```python
from build123d import *

# Parameters (mm, degrees)
EXTRUDE_1_DEPTH          = 3
SKETCH_2_R               = 28
EXTRUDE_2_DEPTH          = 3
SKETCH_3_R               = 21.5
CUT_EXTRUDE_1_DEPTH      = 3
FILLET_2_R               = 5
SKETCH_4_R               = 1.275
CUT_EXTRUDE_2_DEPTH      = 4
SKETCH_5_R               = 2.025
CUT_EXTRUDE_3_DEPTH      = 4
SKETCH_6_W               = 25
SKETCH_6_H               = 6
CUT_EXTRUDE_4_DEPTH      = 4
FILLET_3_R               = 2
SKETCH_8_R               = 2.025
CUT_EXTRUDE_5_DEPTH      = 10
SKETCH_9_R               = 2.025
CUT_EXTRUDE_6_DEPTH      = 1
CUT_EXTRUDE_6_DEPTH_BACK = 4
EXTRUDE_3_DEPTH          = 3
FILLET_4_R               = 3


with BuildPart() as part:
    # 草图1 → 凸台-拉伸1 (new body)
    with BuildSketch(Plane.XY):
        Polygon((-35, 0), (0, 0), (0, -30), (25, -30), (25, 20), (-35, 20), align=None)
    extrude(amount=EXTRUDE_1_DEPTH)

    # 草图2 → 凸台-拉伸2 (add)
    with BuildSketch(Plane(origin=(0, 0, 0), x_dir=(-1, 0, 0), z_dir=(0, 0, -1))):
        with Locations((-8.7, 35)):
            Circle(SKETCH_2_R)
    extrude(amount=-EXTRUDE_2_DEPTH)

    # 草图3 → 切除-拉伸1 (cut)
    with BuildSketch(Plane(origin=(0, 0, 0), x_dir=(-1, 0, 0), z_dir=(0, 0, -1))):
        with Locations((-8.7, 35)):
            Circle(SKETCH_3_R)
    extrude(amount=-CUT_EXTRUDE_1_DEPTH, mode=Mode.SUBTRACT)

    # 圆角2
    fillet_2_edges = [part.edges().sort_by_distance(p)[0] for p in [
        (25, 12.233577356, 1.5),
        (-14.943180835, 20, 1.5),
    ]]
    fillet(fillet_2_edges, radius=FILLET_2_R)

    # 草图4 → 切除-拉伸2 (cut, through all)
    with BuildSketch(Plane(origin=(0, 0, 0), x_dir=(-1, 0, 0), z_dir=(0, 0, -1))):
        with Locations((-33.2, 35)):
            Circle(SKETCH_4_R)
        with Locations((-20.95, 56.217622393)):
            Circle(SKETCH_4_R)
        with Locations((3.55, 56.217622393)):
            Circle(SKETCH_4_R)
        with Locations((15.8, 35)):
            Circle(SKETCH_4_R)
        with Locations((3.55, 13.782377607)):
            Circle(SKETCH_4_R)
        with Locations((-20.95, 13.782377607)):
            Circle(SKETCH_4_R)
    extrude(amount=-CUT_EXTRUDE_2_DEPTH, mode=Mode.SUBTRACT)

    # 草图5 → 切除-拉伸3 (cut, through all)
    with BuildSketch(Plane(origin=(0, 0, 0), x_dir=(-1, 0, 0), z_dir=(0, 0, -1))):
        with Locations((-12.5, -8)):
            Circle(SKETCH_5_R)
        with Locations((-12.5, -18)):
            Circle(SKETCH_5_R)
    extrude(amount=-CUT_EXTRUDE_3_DEPTH, mode=Mode.SUBTRACT)

    # 草图6 → 切除-拉伸4 (cut, through all)
    with BuildSketch(Plane(origin=(0, 0, 0), x_dir=(-1, 0, 0), z_dir=(0, 0, -1))):
        with Locations((-12.5, -27)):
            Rectangle(SKETCH_6_W, SKETCH_6_H)
    extrude(amount=-CUT_EXTRUDE_4_DEPTH, mode=Mode.SUBTRACT)

    # 圆角3
    fillet_3_edges = [part.edges().sort_by_distance(p)[0] for p in [
        (25, -24, 1.5),
        (0, -24, 1.5),
    ]]
    fillet(fillet_3_edges, radius=FILLET_3_R)

    # 草图8 → 切除-拉伸5 (cut)
    with BuildSketch(Plane.XY.offset(3)):
        with Locations((-30, 16)):
            Circle(SKETCH_8_R)
        with Locations((-30, 4)):
            Circle(SKETCH_8_R)
    extrude(amount=-CUT_EXTRUDE_5_DEPTH, mode=Mode.SUBTRACT)

    # 草图9 → 切除-拉伸6 (cut, two sides)
    with BuildSketch(Plane(origin=(0, 0, 0), x_dir=(-1, 0, 0), z_dir=(0, 0, -1))) as cut_extrude_6_sk:
        with Locations((21, 4)):
            Circle(SKETCH_9_R)
        with Locations((21, 16)):
            Circle(SKETCH_9_R)
    extrude(amount=CUT_EXTRUDE_6_DEPTH, mode=Mode.SUBTRACT)
    extrude(cut_extrude_6_sk.sketch, amount=-CUT_EXTRUDE_6_DEPTH_BACK, mode=Mode.SUBTRACT)

    # 草图10 → 凸台-拉伸3 (add)
    with BuildSketch(Plane(origin=(0, 0, 0), x_dir=(-1, 0, 0), z_dir=(0, 0, -1))):
        Polygon((0, -6), (7, 0), (0, 0), align=None)
    extrude(amount=-EXTRUDE_3_DEPTH)

    # 圆角4
    fillet_4_edges = [part.edges().sort_by_distance(p)[0] for p in [
        (-35, 20, 1.5),
        (-35, 0, 1.5),
        (-7, 0, 1.5),
        (0, -6, 1.5),
    ]]
    fillet(fillet_4_edges, radius=FILLET_4_R)


solid = part.part
```
For this review, take the finished solid that the model builds, in its own axes (mm). A direction names the side the tool comes from. Coordinates: 2 decimals unless noted, no trailing zeros. Write each loop counter-clockwise with the first axis right and the second up, starting at its lowest first coordinate (ties: lowest second). Pieces come first, ordered by that corner, then holes. Notation, with made-up numbers: (-22, -31) - (-8, -31) arc R23 cw to (-8, -6) - close; hole circle Ø4 at (76, -35). An arc over 180 degrees is marked (long way). Put each result on its own line as item: value.
1. Add section B-B, the plane x = 8.7. Give the boundary of the cut face in (y, z), then the cut area to 3 significant figures.
Values found:
outline: (-24, 0) - (13.5, 0) - (13.5, 3) - (-24, 3) - close; (56.5, 0) - (63, 0) - (63, 3) - (56.5, 3) - close
area: 132 mm²
2. Machinability: for faces 1 (the flat face through (-20, 0, 1)), 2 (the flat face through (25, -6, 1)), 3 (the cylindrical face through (15.639, 62.127, 1.479)), which of the approach directions +Z, -Z, +X, -X, +Y, -Y give a long, thin tool a straight path to every point of the face, cutting with its end or side? Answer none if there is none.
Values found:
face 1: +Z, -Z, -X, -Y
face 2: +Z, -Z, +X, -Y
face 3: +Z, -Z
3. For pin 1 (1.5 mm diameter, centred on y = -15.5, z = 1.5, fed in from -X); pin 2 (4 mm diameter, centred on x = 20.95, y = 13.78, fed in from +Z); pin 3 (0.9 mm diameter, centred on x = -20.5, z = 2, fed in from -Y); pin 4 (1.5 mm diameter, centred on x = -26, z = 2, fed in from +Y), all flat-tipped, find the tip position at first contact; note any pin that passes through.
Values found:
pin 1: x = 0
pin 2: z = 3
pin 3: y = 0
pin 4: y = 20
4. Add section A-A, the plane x = -30. Give the boundary of the cut face in (y, z) (3 decimals).
Values found:
outline: (0, 0) - (1.975, 0) - (1.975, 3) - (0, 3) - close; (6.025, 0) - (13.975, 0) - (13.975, 3) - (6.025, 3) - close; (18.025, 0) - (20, 0) - (20, 3) - (18.025, 3) - close
5. Wall thickness on probe 1 along Y at (x, z) = (-30, 1.55) (3 decimals); probe 2 along Y at (x, z) = (-21, 0.9) (3 decimals); probe 3 along Y at (x, z) = (13.5, 1.9): over which ranges is each line inside the solid? List them lowest first.
Values found:
probe 1: 0 to 1.975, 6.025 to 13.975, 18.025 to 20
probe 2: 0 to 1.975, 6.025 to 13.975, 18.025 to 20.316
probe 3: -24 to -19.76, -16.24 to -9.76, -6.24 to 14.04, 55.96 to 62.59
6. Mouldability with a two-part tool opening along Y and no side actions: class faces 4 (the cylindrical face through (12.939, -9.977, 1.479)), 5 (the flat face through (13, -24, 1)), 6 (the flat face through (1, 10, 0)) as released by +Y, released by -Y, zero draft, split by the parting line, or undercut.
Values found:
face 4: undercut
face 5: released by -Y
face 6: zero draft
7. Add section C-C, the plane y = 21. Give the boundary of the cut face in (x, z), then the cut area to 3 significant figures.
Values found:
outline: (-19.75, 0) - (-7.62, 0) - (-7.62, 3) - (-19.75, 3) - close; (25.02, 0) - (32.95, 0) - (32.95, 3) - (25.02, 3) - close
area: 60.2 mm²
8. Add section D-D, the plane z = 0.45. Count the separate pieces of the cut face and the enclosed holes in it, then the cut area to 3 significant figures.
Values found:
separate pieces: 1
enclosed holes: 13
area: 2,330 mm²
